Input: dimensioned drawing with shaded views. Units: mm. Origin: part minimum x, y, z. A direction names the side the tool comes from. Give positions to 0.01 mm unless a question says otherwise; leave off trailing zeros. Loops run counter-clockwise (first coordinate to the right, second up) from the corner with the lowest first, then second, coordinate; pieces in that order, holes last.
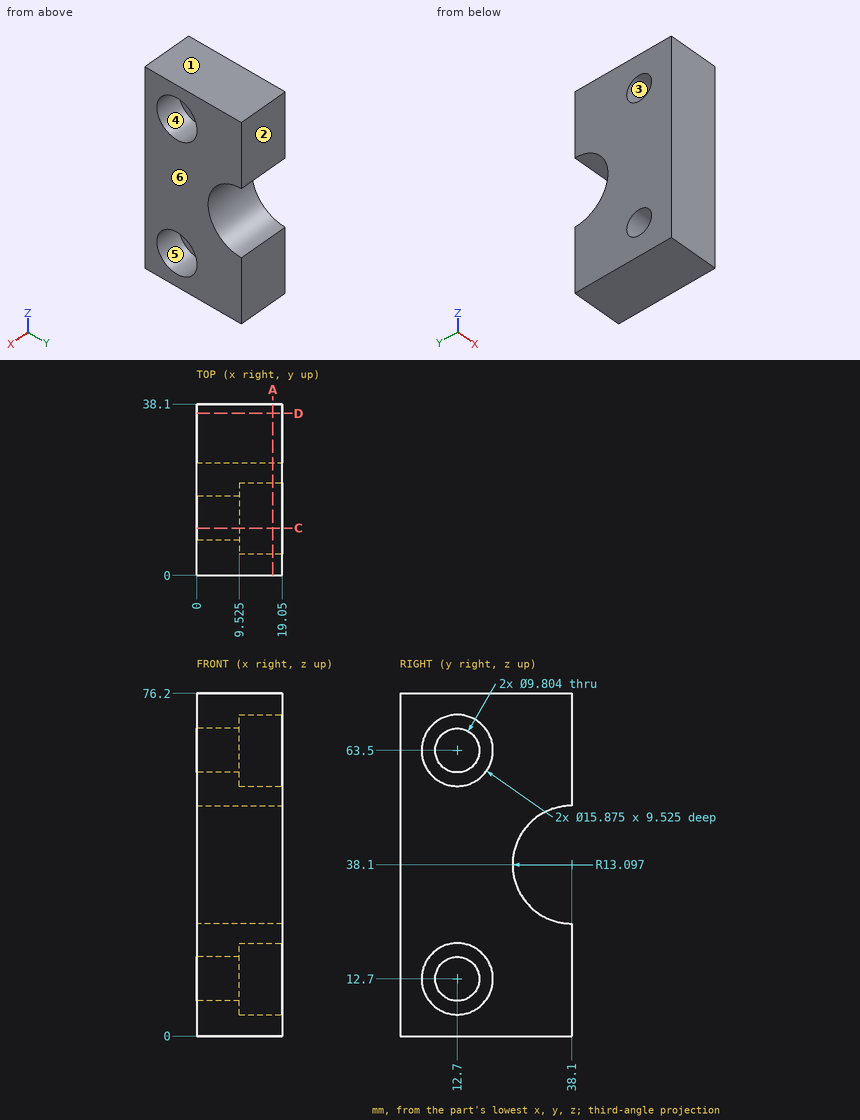
(1) First-contact query: pin 1 (14.5 mm diameter, centred on y = 12.7, z = 63.5, fed in from +X) (3 decimals). Flat tip, straight axial feed; report the tip coordinate or a pass-through.
A:
pin 1: stops at x = 9.525
(2) Section A-A, the plane x = 17. Return the cut outline in (y, z) (1 decimal), then the cut area to 3 significant figures.
A:
outline: (0, 0) - (38.1, 0) - (38.1, 25) arc R13.1 cw to (38.1, 51.2) - (38.1, 76.2) - (0, 76.2) - close; hole circle Ø15.9 at (12.7, 12.7); hole circle Ø15.9 at (12.7, 63.5)
area: 2,240 mm2
(3) Reachability of the marked faces 5 and 6 from +Z, -Z, +X, -X, +Y, -Y: full face, straight path, thin tool, end or side. Return the list, or none.
A:
face 5: +X
face 6: +Z, -Z, +X, +Y, -Y
(4) Section C-C, the plane y = 10.5. Count the separate pieces of the cut face and the enclosed holes in it, then the cut area to 3 significant figures.
A:
separate pieces: 3
enclosed holes: 0
area: 994 mm2
(5) Mould query, pull axis Y, two halves, no side actions, for the marked faces 1, 2, 3 and 4. Classes: pulls with the +Y half, pulls with the -Y half, needs draft (parallel to the pull), parting line crosses it, or undercut.
A:
face 1: needs draft
face 2: pulls with the +Y half
face 3: undercut
face 4: undercut
(6) Section D-D, the plane y = 36. Return the cut outline in (x, z), then the cut area to 3 significant figures.
A:
outline: (0, 0) - (19.05, 0) - (19.05, 25.17) - (0, 25.17) - close; (0, 51.03) - (19.05, 51.03) - (19.05, 76.2) - (0, 76.2) - close
area: 959 mm2
(7) Ray query, line 1 along Z through (x, y) = (10, 6.5) (1 decimal); line 2 along Z through (x, y) = (2, 11); line 3 along Y through (x, z) = (17, 19.5) (1 decimal). Return the intervals inside material, ascending.
A:
line 1: z = 0 to 7.7, 17.7 to 58.5, 68.5 to 76.2
line 2: z = 0 to 8.1, 17.3 to 58.9, 68.1 to 76.2
line 3: y = 0 to 8.6, 16.8 to 38.1
